```python
from build123d import *

# Parameters (mm, degrees)
F1_DEPTH = 10


with BuildPart() as f1:
    # F0 (on Top) → F1 (new body)
    with BuildSketch(Plane.XY):
        with BuildLine():
            ThreePointArc((0.202041, 23), (0.151403, 24.00509), (0, 25))
            ThreePointArc((0, 25), (-5, 24.494897), (-9.797959, 23))
            ThreePointArc((-9.797959, 23), (-7.485281, 18.36897), (-3.166929, 15.514719))
            ThreePointArc((-3.166929, 15.514719), (-0.679014, 18.895752), (0.202041, 23))
        make_face()
        with BuildLine():
            ThreePointArc((-18.028245, 17.32), (-9.335253, -23.191659), (25, 0))
            ThreePointArc((25, 0), (20.856042, 13.784974), (9.797959, 23))
            ThreePointArc((9.797959, 23), (5, 16.339746), (-3.166929, 15.514719))
            ThreePointArc((-3.166929, 15.514719), (-11.003846, 13.072974), (-18.028245, 17.32))
        make_face()
        with BuildLine():
            ThreePointArc((-9.797959, 23), (-14.2, 20.575714), (-18.028245, 17.32))
            ThreePointArc((-18.028245, 17.32), (-11.003846, 13.072974), (-3.166929, 15.514719))
            ThreePointArc((-3.166929, 15.514719), (-7.485281, 18.36897), (-9.797959, 23))
        make_face()
        with BuildLine():
            ThreePointArc((-3.166929, 15.514719), (5, 16.339746), (9.797959, 23))
            ThreePointArc((9.797959, 23), (5, 24.494897), (0, 25))
            ThreePointArc((0, 25), (0.151403, 24.00509), (0.202041, 23))
            ThreePointArc((0.202041, 23), (-0.679014, 18.895752), (-3.166929, 15.514719))
        make_face()
    extrude(amount=F1_DEPTH)


solid = f1.part
```
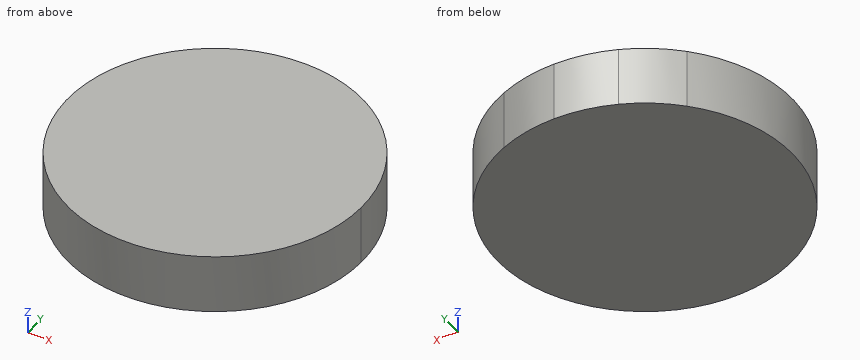
Verification items for the finished model (mm, model axes). Coordinates: 2 decimals unless noted, no trailing zeros. Order: outer loops, then holes, each group sorted by start corner. A loop starts at its lowest first (then second) coordinate and runs counter-clockwise, first axis right, second up. Notation, with made-up numbers: (8.5, 55) -> (32.5, 55) arc R17 ccw to (32.5, 80) -> close; hole circle Ø6 at (-1, 29). An arc over 180 degrees is marked (long way). Answer as CSV lines item,"result". Start each with the question number.
1) Gauge pin test, flat ends, axial feed: pin 1 Ø1 at (x, z) = (-4, 3) entering from -Y; pin 2 Ø4 at (y, z) = (19, 4.5) entering from -X; pin 3 Ø3 at (y, z) = (-6.5, 7.5) entering from -X. Record the tip position at first contact, or that the pin passes through.
2) Cross-section at B-B, the plane y = -11. Record the boundary of the cut face in (x, z), then the cut area to 3 significant figures.
3) Cross-section at A-A, the plane z = 2. Record the boundary of the cut face in (x, y).
4) Material ranges on L1, parallel to Y at x = 19, z = 7.75; L2, parallel to Y at x = 17, z = 5.5; L3, parallel to X at y = 4, z = 1.25, recorded low to high. Write a range as [from, to].
Conclusion:
1,pin 1,"stops at y = -24.75"
1,pin 2,"stops at x = -18.33"
1,pin 3,"stops at x = -24.49"
2,outline,"(-22.45, 0) -> (22.45, 0) -> (22.45, 10) -> (-22.45, 10) -> close"
2,area,"449 mm²"
3,outline,"(-18.03, 17.32) arc R25 ccw (long way) to (9.8, 23) arc R25 ccw to (0, 25) arc R25 ccw to (-9.8, 23) arc R25 ccw to start"
4,L1,"y = [-16.25, 16.25]"
4,L2,"y = [-18.33, 18.33]"
4,L3,"x = [-24.68, 24.68]"
